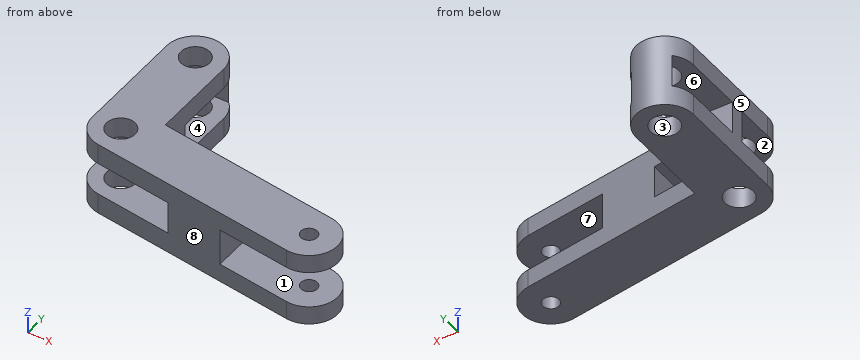
```python
from build123d import *

# Parameters (mm, degrees)
SKETCH_1_R          = 1.75
SKETCH_1_R_2        = 1
EXTRUDE_1_DEPTH     = 4.5
SKETCH_5_W          = 9.199682462
SKETCH_5_H          = 9.813167506
SKETCH_5_W_2        = 14.660354758
SKETCH_5_H_2        = 10.525453646
CUT_EXTRUDE_3_DEPTH = 2
SKETCH_6_W          = 19.186818514
SKETCH_6_H          = 12
CUT_EXTRUDE_4_DEPTH = 2.25


with BuildPart() as part:
    # 草图1 → 凸台-拉伸1 (new, symmetric)
    with BuildSketch(Plane.XY):
        with BuildLine():
            Line((25.152003619, -7.458331848), (-0.538461538, -3.458331848))
            ThreePointArc((-0.538461538, -3.458331848), (-2.658440839, -2.276552725), (-3.5, 0))
            Line((-3.5, 0), (-3.5, 14))
            ThreePointArc((-3.5, 14), (0, 17.5), (3.5, 14))
            Line((3.5, 14), (3.5, 2.997220935))
            Line((3.5, 2.997220935), (26.228926696, -0.541668152))
            ThreePointArc((26.228926696, -0.541668152), (29.148797005, -4.538461538), (25.152003619, -7.458331848))
        make_face()
        Circle(SKETCH_1_R, mode=Mode.SUBTRACT)
        with Locations((0, 14)):
            Circle(SKETCH_1_R, mode=Mode.SUBTRACT)
        with Locations((25.690465157, -4)):
            Circle(SKETCH_1_R_2, mode=Mode.SUBTRACT)
    extrude(amount=EXTRUDE_1_DEPTH, both=True)

    # 草图5 → 切除-拉伸3 (cut, symmetric)
    with BuildSketch(Plane.XY):
        with Locations((-1.099841231, 11.563279791)):
            Rectangle(SKETCH_5_W, SKETCH_5_H)
        with Locations((1.684655549, -0.393377614)):
            Rectangle(SKETCH_5_W_2, SKETCH_5_H_2)
    extrude(amount=CUT_EXTRUDE_3_DEPTH, both=True, mode=Mode.SUBTRACT)

    # 草图6 → 切除-拉伸4 (cut, symmetric)
    with BuildSketch(Plane.XY):
        with Locations((25.690465157, -4)):
            Rectangle(SKETCH_6_W, SKETCH_6_H)
    extrude(amount=CUT_EXTRUDE_4_DEPTH, both=True, mode=Mode.SUBTRACT)


solid = part.part
```
The listing builds one solid part. Answer for the finished solid, in the listing's coordinates (mm). Face numbers are marked on the shaded views. A direction names the side the tool comes from. Give positions to 0.01 mm unless a question says otherwise; leave off trailing zeros. Order: outer loops, then holes, each group sorted by start corner. A loop starts at its lowest first (then second) coordinate and runs counter-clockwise, first axis right, second up. Notation, with made-up numbers: (-7.5, 63) - (15.5, 63) arc R25 cw to (15.5, 93) - close; hole circle Ø2 at (30.25, 46.5). An arc over 180 degrees is marked (long way). Answer in a Markdown table with one row per item. Add a question column.
Q1. The part is cut by section C-C (x = 0). Determine the outline of the cut face in (y, z).
Q2. Find the intervals of material crossed by line 1 along Z through (x, y) = (-0.5, 10.25); line 2 along Z through (x, y) = (22, -0.75); line 3 along X through (y, z) = (14, 3.45), in increasing order. Write a range as [from, to].
Q3. Which of the six approach directions +Z, -Z, +X, -X, +Y, -Y give full straight-line access (tool end or side, diameter ignored) to the marked faces 1, 2, 3, 4 and 5?
Q4. The part is cut by section A-A (y = 11). Determine the outline of the cut face in (x, z).
Q5. The part is cut by section B-B (z = 0.5). Determine the outline of the cut face in (x, y).
Q6. For a pull along Y with two mould halves and no side action, classify the marked faces 6, 7 and 8 as released by +Y, released by -Y, zero draft, split by the parting line, or undercut.
Q7. Given P1, Ø10, axis at x = 5.5, y = 13, coming from the +Z side; P2, Ø4.5, axis at x = -0.5, z = 1, coming from the -Y side; P3, Ø4, axis at y = 0, z = -3.5, coming from the +X side; P4, Ø1.2, axis at y = -2.5, z = 0, coming from the -X side, each flat-ended and moving along its own axis, determine where each tip first touches the part or whether it passes through.
Q8. The part is cut by section D-D (y = -4.5). Determine the outline of the cut face in (x, z), then the cut area to 3 significant figures.
Determined:
| question | item | result |
|---|---|---|
| 1 | outline | (-3.54, -4.5) - (-1.75, -4.5) - (-1.75, -2) - (-3.54, -2) - close; (-3.54, 2) - (-1.75, 2) - (-1.75, 4.5) - (-3.54, 4.5) - close; (1.75, -4.5) - (12.25, -4.5) - (12.25, -2) - (6.66, -2) - (6.66, 2) - (12.25, 2) - (12.25, 4.5) - (1.75, 4.5) - (1.75, 2) - (4.87, 2) - (4.87, -2) - (1.75, -2) - close; (15.75, -4.5) - (17.5, -4.5) - (17.5, 4.5) - (15.75, 4.5) - (15.75, 2) - (16.47, 2) - (16.47, -2) - (15.75, -2) - close |
| 2 | line 1 | z = [-4.5, -2], [2, 4.5] |
| 2 | line 2 | z = [-4.5, -2.25], [2.25, 4.5] |
| 2 | line 3 | x = [-3.5, -1.75], [1.75, 3.5] |
| 3 | face 1 | +X, +Y, -Y |
| 3 | face 2 | -X, -Y |
| 3 | face 3 | +Z, -Z |
| 3 | face 4 | +X, -X |
| 3 | face 5 | +Z, -Z, -X, +Y, -Y |
| 4 | outline | (-3.5, -4.5) - (3.5, -4.5) - (3.5, -2) - (-3.5, -2) - close; (-3.5, 2) - (3.5, 2) - (3.5, 4.5) - (-3.5, 4.5) - close |
| 5 | outline | (-3.5, 4.87) - (3.5, 4.87) - (3.5, 6.66) - (-3.5, 6.66) - close; (-2.48, 16.47) - (2.48, 16.47) arc R3.5 ccw to start; (9.01, -4.95) - (16.1, -6.05) - (16.1, 1.04) - (9.01, 2.14) - close |
| 6 | face 6 | undercut |
| 6 | face 7 | zero draft |
| 6 | face 8 | released by -Y |
| 7 | P1 | stops at z = 4.5 |
| 7 | P2 | stops at y = -3.78 |
| 7 | P3 | stops at x = 28.56 |
| 7 | P4 | stops at x = 9.01 |
| 8 | outline | (6.15, -4.5) - (24.82, -4.5) - (24.82, -2.25) - (16.1, -2.25) - (16.1, 2.25) - (24.82, 2.25) - (24.82, 4.5) - (6.15, 4.5) - (6.15, 2) - (9.01, 2) - (9.01, -2) - (6.15, -2) - close; (26.56, -4.5) - (29.15, -4.5) - (29.15, -2.25) - (26.56, -2.25) - close; (26.56, 2.25) - (29.15, 2.25) - (29.15, 4.5) - (26.56, 4.5) - close |
| 8 | area | 129 mm² |
